For this review, use the dimensioned drawing (mm, ordinates from the lowest corner) and the shaded views. A direction names the side the tool comes from. Give positions to 0.01 mm unless a question says otherwise; leave off trailing zeros. Write each loop counter-clockwise with the first axis right and the second up, starting at its lowest first coordinate (ties: lowest second). Pieces come first, ordered by that corner, then holes. Notation, with made-up numbers: (89.5, 69) -> (112.5, 69) arc R35 cw to (112.5, 102) -> close; hole circle Ø6 at (68.25, 89.25). An arc over 180 degrees is marked (long way). Return JSON: item names as keys, results as strings.
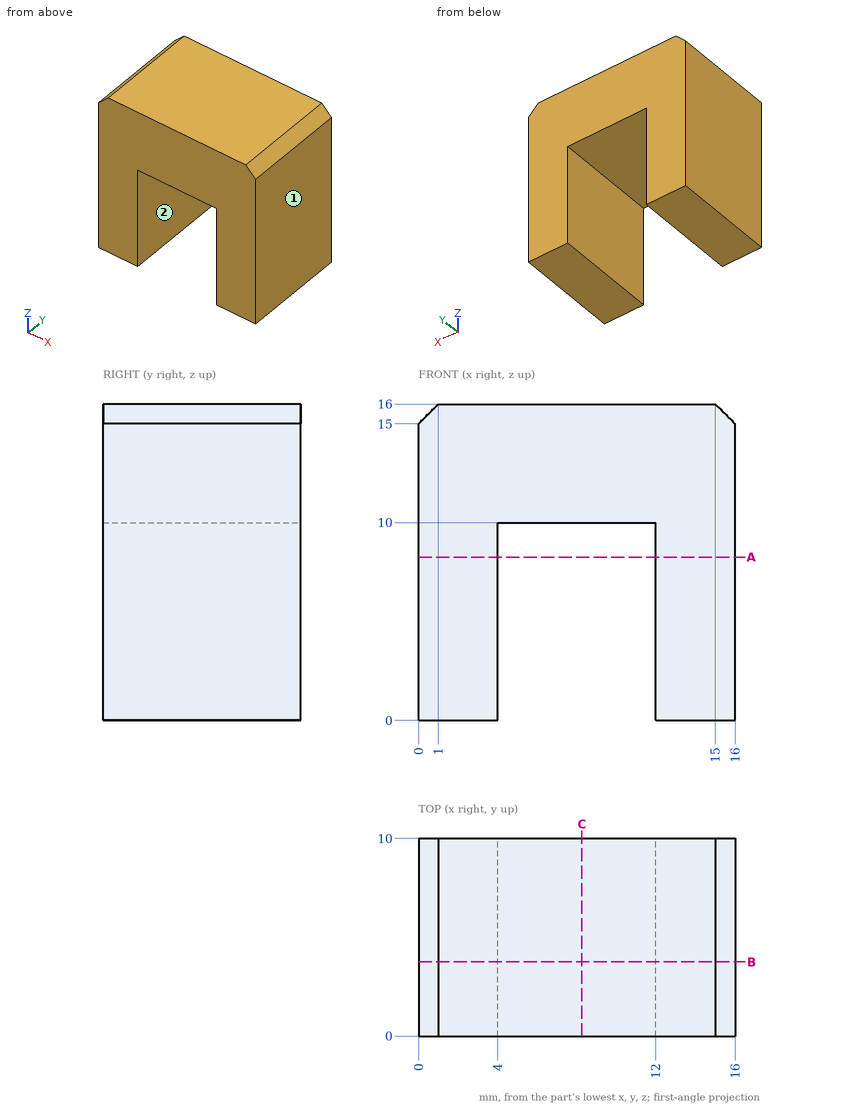
1. Add section A-A, the plane z = 8.25. State the section outline as (x, y) points.
Results found:
{"outline": "(0, 0) -> (4, 0) -> (4, 10) -> (0, 10) -> close; (12, 0) -> (16, 0) -> (16, 10) -> (12, 10) -> close"}
2. Add section B-B, the plane y = 3.75. State the section outline as (x, z) points.
Results found:
{"outline": "(0, 0) -> (4, 0) -> (4, 10) -> (12, 10) -> (12, 0) -> (16, 0) -> (16, 15) -> (15, 16) -> (1, 16) -> (0, 15) -> close"}
3. For the marked faces 1 and 2, list the 3-axis set-ups (+Z, -Z, +X, -X, +Y, -Y) from which the entire face can be reached by the end or side of a thin tool; tool diameter is ignored.
Results found:
{"face 1": "+Z, -Z, +X, +Y, -Y", "face 2": "-Z, +Y, -Y"}
4. Add section C-C, the plane x = 8.25. State the section outline as (y, z) points.
Results found:
{"outline": "(0, 10) -> (10, 10) -> (10, 16) -> (0, 16) -> close"}
5. To check wall thickness, follow probe 1 along X at (y, z) = (8, 7.75); probe 2 along Z at (x, y) = (11, 0.5); probe 3 along Z at (x, y) = (15.25, 4.5). State the ranges of each line that lie inside material, in increasing order.
Results found:
{"probe 1": "x = 0 to 4, 12 to 16", "probe 2": "z = 10 to 16", "probe 3": "z = 0 to 15.75"}
